The model under review builds one solid part; all positions refer to its coordinate system, in mm. A direction names the side the tool comes from. Round coordinates to 2 decimals unless told otherwise and drop trailing zeros. Loops run counter-clockwise (first coordinate to the right, second up) from the corner with the lowest first, then second, coordinate; pieces in that order, holes last. Notation, with made-up numbers: (73.25, 76.5) -> (124.25, 76.5) arc R31 cw to (124.25, 102.5) -> close; hole circle Ø4 at (-5.5, 85.5). An arc over 180 degrees is marked (long way). Use a Markdown table: item, result. Add a question column.
1) Wall thickness on probe 1 along Z at (x, y) = (3.25, 98); probe 2 along Y at (x, z) = (-1.5, -5.25); probe 3 along X at (y, z) = (52.5, -5): over which ranges is each line inside the solid? List them lowest first.
2) Consider section C-C on y = 6. Give the boundary of the cut face in (x, z).
3) Consider section B-B on z = -6. Give the boundary of the cut face in (x, y), plus the area to 3 significant figures.
4) For faces 1 (the flat face through (0, 99, -2)), 2 (the flat face through (0, 90, 6)), 3 (the flat face through (0, 98, -0.5)), list the 3-axis set-ups (+Z, -Z, +X, -X, +Y, -Y) from which the entire face can be reached by the end or side of a thin tool; tool diameter is ignored.
5) Consider section D-D on x = -4. Give the boundary of the cut face in (y, z), plus the area to 3 significant figures.
6) Insertion check: pin 1 (0.5 mm diameter, centred on x = 1, z = 0, fed in from +Y); pin 2 (8 mm diameter, centred on x = -1, z = 3, fed in from -Y); pin 3 (1.5 mm diameter, centred on y = 86.5, z = 4.5, fed in from -X); pin 4 (6 mm diameter, centred on x = 3.5, y = 96.5, fed in from -Z). Each pin has a flat end and moves straight along its axis. Give the tip position at first contact, or say it passes through.
7) Consider section A-A on x = 0. Give the boundary of the cut face in (y, z).
Autodesk Inventor part; units mm, degrees
ref_plane "YZ Plane" through (0, 0, 0) normal (1, 0, 0) x (0, 1, 0)
ref_plane "XZ Plane" through (0, 0, 0) normal (0, 1, 0) x (-1, 0, 0)
ref_plane "XY Plane" through (0, 0, 0) normal (0, 0, 1) x (1, 0, 0)
sketch "Sketch1" plane through (0, 0, 0) normal (0, 1, 0) x (-1, 0, 0)
  line L0 (0, -10.5) -> (0, 10.5)
  line L1 (-10.5, 0) -> (10.5, 0)
  circle A0 centre (0, 0) radius 7.5
  dimension "d0" = 15
extrude "Extrusion1" add sketch "Sketch1" along normal blind 90
sketch "Sketch2" plane through (0, 90, 0) normal (0, 1, 0) x (1, 0, 0)
  line L0 (10.5, 0) -> (-10.5, 0)
  line L1 (0, 10.5) -> (0, -10.5)
  line L2 (-7.2284, 2) -> (7.2284, 2)
  line L3 (-7.2284, -2) -> (7.2284, -2)
  circle A0 centre (0, 0) radius 7.5
  arc A1 (7.2284, -2) -> (7.2284, 2) centre (0, 0) ccw
  arc A2 (-7.2284, 2) -> (-7.2284, -2) centre (0, 0) ccw
  point P0 (7.2284, -2)
  dimension "d3" = 4
  dimension "d4" = 15
  dimension "d5" = 4
extrude "Extrusion2" add sketch "Sketch2" along normal blind 15 contours A0 L3 L1 L0 | L0 L1 L2 A0 | L1 L3 A0 L0 | L0 A0 L2 L1
fillet "Fillet1" radius 3 2 edges at (0, 90, 2) (0, 90, -2)
sketch "Sketch3" plane through (0, 105, 0) normal (0, 1, 0) x (1, 0, 0)
  line L0 (-7.2284, -2) -> (7.2284, -2)
  line L1 (7.2284, 2) -> (-7.2284, 2)
  arc A0 (7.2284, -2) -> (7.2284, 2) centre (0, 0) ccw
  arc A1 (-7.2284, 2) -> (-7.2284, -2) centre (0, 0) ccw
  line L2 (-5.9791, 0.5) -> (5.9791, 0.5)
  arc A2 (5.9791, -0.5) -> (5.9791, 0.5) centre (0, 0) ccw
  line L3 (5.9791, -0.5) -> (-5.9791, -0.5)
  arc A3 (-5.9791, 0.5) -> (-5.9791, -0.5) centre (0, 0) ccw
  dimension "d9" = 1.5
extrude "Extrusion3" cut sketch "Sketch3" against normal blind 15 contours L2 A2 L3 A3
fillet "Fillet2" radius 2 2 edges at (7.5, 105, 0) (-7.5, 105, 0)
properties part number "PUFIK_2"
Result set:
| question | item | result |
|---|---|---|
| 1 | probe 1 | -2 to -0.5, 0.5 to 2 |
| 1 | probe 2 | 0 to 90 |
| 1 | probe 3 | -5.59 to 5.59 |
| 2 | outline | circle Ø15 at (0, 0) |
| 3 | outline | (-4.5, 0) -> (4.5, 0) -> (4.5, 90) -> (-4.5, 90) -> close |
| 3 | area | 810 mm2 |
| 4 | face 1 | -Z, +X, -X, +Y |
| 4 | face 2 | +Z, +X, -X, +Y |
| 4 | face 3 | +Y |
| 5 | outline | (0, -6.34) -> (90, -6.34) -> (90, -5) arc R3 cw to (93, -2) -> (105, -2) -> (105, -0.5) -> (90, -0.5) -> (90, 0.5) -> (105, 0.5) -> (105, 2) -> (93, 2) arc R3 cw to (90, 5) -> (90, 6.34) -> (0, 6.34) -> close |
| 5 | area | 1,190 mm2 |
| 6 | pin 1 | y = 90 |
| 6 | pin 2 | y = 0 |
| 6 | pin 3 | x = -6.5 |
| 6 | pin 4 | z = -2 |
| 7 | outline | (0, -7.5) -> (90, -7.5) -> (90, -5) arc R3 cw to (93, -2) -> (105, -2) -> (105, -0.5) -> (90, -0.5) -> (90, 0.5) -> (105, 0.5) -> (105, 2) -> (93, 2) arc R3 cw to (90, 5) -> (90, 7.5) -> (0, 7.5) -> close |
